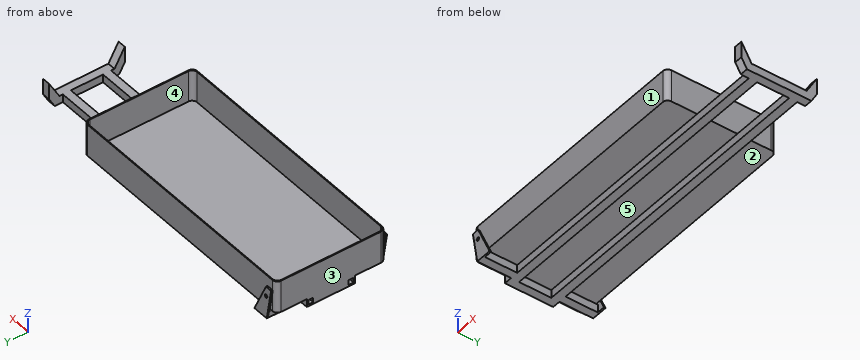
```python
from build123d import *

# Parameters (mm, degrees)
F0_W          = 990.6
F0_H          = 127
F1_DEPTH      = 431.8
F2_R          = 19.05
F4_DEPTH      = 123.825
F5_W          = 31.75
F5_H          = 31.75
F5_W_2        = 19.05
F5_H_2        = 19.05
F6_DEPTH      = 762
F6_DEPTH_BACK = 495.3
F7_W          = 31.75
F7_H          = 31.75
F7_W_2        = 19.0499997139
F7_H_2        = 19.0499997139
F8_DEPTH      = 127
F10_W         = 31.75
F10_H         = 31.75
F10_W_2       = 19.05
F10_H_2       = 19.05
F11_DEPTH     = 127
F12_W         = 31.75
F12_H         = 31.75
F12_W_2       = 19.0499814987
F12_H_2       = 19.0499814987
F13_DEPTH     = 127
F15_R         = 6.35
F16_DEPTH     = 6.35
F18_R         = 6.35
F19_DEPTH     = 6.35
F22_DEPTH     = 31.75


with BuildPart() as f1:
    # F0 (on Front) → F1 (new body)
    with BuildSketch(Plane.XZ):
        Rectangle(F0_W, F0_H)
    extrude(amount=F1_DEPTH)

    # F2
    f2_edges = [f1.edges().sort_by_distance(p)[0] for p in [
        (495.3, -431.8, 0),
        (495.3, 0, 0),
        (-495.3, -431.8, 0),
        (-495.3, 0, 0),
    ]]
    fillet(f2_edges, radius=F2_R)

    # F3 (on face) → F4 (cut)
    with BuildSketch(Plane.XY.offset(63.5)):
        with BuildLine():
            ThreePointArc((492.125, -22.225), (486.5453841816, -8.7546158184), (473.075, -3.175))
            Line((473.075, -3.175), (-473.075, -3.175))
            ThreePointArc((-473.075, -3.175), (-486.5453841816, -8.7546158184), (-492.125, -22.225))
            Line((-492.125, -22.225), (-492.125, -409.575))
            ThreePointArc((-492.125, -409.575), (-486.5453841816, -423.0453841816), (-473.075, -428.625))
            Line((-473.075, -428.625), (473.075, -428.625))
            ThreePointArc((473.075, -428.625), (486.5453841816, -423.0453841816), (492.125, -409.575))
            Line((492.125, -409.575), (492.125, -22.225))
        make_face()
    extrude(amount=-F4_DEPTH, mode=Mode.SUBTRACT)

    # F5 (on Right) → F6 (join, two sides)
    with BuildSketch(Plane.YZ) as f6_sk:
        with Locations((-295.275, -79.375)):
            Rectangle(F5_W, F5_H)
        with Locations((-295.275, -79.375)):
            Rectangle(F5_W_2, F5_H_2, mode=Mode.SUBTRACT)
        with Locations((-136.525, -79.375)):
            Rectangle(F5_W, F5_H)
        with Locations((-136.525, -79.375)):
            Rectangle(F5_W_2, F5_H_2, mode=Mode.SUBTRACT)
    extrude(amount=F6_DEPTH)
    extrude(f6_sk.sketch, amount=-F6_DEPTH_BACK)

    # F7 (on face) → F8 (join)
    with BuildSketch(Plane.XZ.offset(152.4)):
        with Locations((-479.425, -79.375)):
            Rectangle(F7_W, F7_H)
        with Locations((-479.425, -79.375)):
            Rectangle(F7_W_2, F7_H_2, mode=Mode.SUBTRACT)
    extrude(amount=F8_DEPTH)

    # F10 (on face) → F11 (join)
    with BuildSketch(Plane.XZ.offset(311.15)):
        with Locations((-447.675, -79.375)):
            Rectangle(F10_W, F10_H)
        with Locations((-447.675, -79.375)):
            Rectangle(F10_W_2, F10_H_2, mode=Mode.SUBTRACT)
    extrude(amount=F11_DEPTH)

    # F12 (on face) → F13 (join)
    with BuildSketch(Plane(origin=(0, -120.65, 0), x_dir=(-1, 0, 0), z_dir=(0, 1, 0))):
        with Locations((447.675, -79.375)):
            Rectangle(F12_W, F12_H)
        with Locations((447.675, -79.375)):
            Rectangle(F12_W_2, F12_H_2, mode=Mode.SUBTRACT)
    extrude(amount=F13_DEPTH)

    # F15 (on offset) → F16 (join)
    with BuildSketch(Plane.XZ.offset(438.15)):
        with BuildLine():
            Line((-485.2864735093, 28.0236670359), (-463.55, -95.25))
            Line((-463.55, -95.25), (-405.0337517073, -95.25))
            ThreePointArc((-405.0337517073, -95.25), (-402.3559838669, -93.7809262565), (-402.1562244835, -90.733187019))
            Line((-402.1562244835, -90.733187019), (-458.4162434399, 29.916812981))
            ThreePointArc((-458.4162434399, 29.916812981), (-459.5878444072, 31.2527678405), (-461.2937706637, 31.75))
            Line((-461.2937706637, 31.75), (-482.1597088935, 31.75))
            ThreePointArc((-482.1597088935, 31.75), (-484.5919000004, 30.6158506608), (-485.2864735093, 28.0236670359))
        make_face()
        with Locations((-459.8815916286, -6.35)):
            Circle(F15_R, mode=Mode.SUBTRACT)
    extrude(amount=F16_DEPTH)

    # F18 (on offset) → F19 (join)
    with BuildSketch(Plane(origin=(0, 6.35, 0), x_dir=(-1, 0, 0), z_dir=(0, 1, 0))):
        Polygon((400.05, -95.25), (463.55, -95.25), (485.94352655, 31.75), (459.2710725857, 31.75), align=None)
        with Locations((459.8815916286, -6.35)):
            Circle(F18_R, mode=Mode.SUBTRACT)
    extrude(amount=F19_DEPTH)

    # F21 (on offset) → F22 (join)
    with BuildSketch(Plane.YZ.offset(762)):
        Polygon((-324.5691289532, -63.5), (-364.8970452561, 6.35), (-364.8970452561, -57.15), (-342.9, -95.25), (-88.9, -95.25), (-66.9029547439, -57.15), (-66.9029547439, 6.35), (-107.2308710468, -63.5), align=None)
    extrude(amount=F22_DEPTH)


solid = f1.part
```
Could you check a few things on this model? Use its own coordinates, in mm. Face numbers are marked on the shaded views. A direction names the side the tool comes from. Coordinates: 2 decimals unless noted, no trailing zeros. Order: outer loops, then holes, each group sorted by start corner. A loop starts at its lowest first (then second) coordinate and runs counter-clockwise, first axis right, second up. Notation, with made-up numbers: M -20,66.5 L -10,66.5 A10 cw -10,70.5 Z; hole C 42,19 d11. An arc over 180 degrees is marked long. Use a Markdown table: item, result. Add a question column.
Q1. Which directions (+Z, -Z, +X, -X, +Y, -Y) give clear straight access to the entire face, cutting with the end or side of a thin tool? Please do the marked faces 4 and 5.
Q2. If I drill on L1, parallel to X at y = -84, z = -39.5 (3 decimals); L2, parallel to Y at x = 400, z = 39 (3 decimals); L3, parallel to Z at x = 46.5, y = -299 (3 decimals), over which ranges is the centre line in solid material (lowest first)?
Q3. I want a section at D-D on z = 46.5. List the corners of the cut face in (x, y) for me (3 decimals).
Q4. I want a section at B-B on y = -170.5. List the corners of the cut face in (x, z) for me (3 decimals), then the cut area to 3 significant figures.
Q5. We'd pull the mould along X, two halves only. Please class the marked faces 1, 2 and 3: pulls with the +X half, pulls with the -X half, needs draft (parallel to the pull), parting line crosses it, or undercut.
Q6. I want a section at A-A on x = 597.5. List the corners of the cut face in (y, z) for me.
Q7. I'm going to push flat-ended pins straight in: pin 1 (1 mm diameter, centred on x = 464.5, y = -230, fed in from +Z) (3 decimals); pin 2 (12 mm diameter, centred on x = -188.5, z = -19, fed in from +Y); pin 3 (9.5 mm diameter, centred on x = 387, z = -75, fed in from +Y). Where does each tip first touch, or does it pass through?
Q8. I want a section at C-C on x = 69.5. List the corners of the cut face in (y, z) for me (3 decimals).
Checked values:
| question | item | result |
|---|---|---|
| 1 | face 4 | +Z |
| 1 | face 5 | -Z |
| 2 | L1 | -495.3 to -492.125, 492.125 to 495.3, 762 to 793.75 |
| 2 | L2 | -431.8 to -428.625, -3.175 to 0 |
| 2 | L3 | -95.25 to -88.9, -69.85 to -60.325 |
| 3 | outline | M -495.3,-412.75 A19.05 ccw -476.25,-431.8 L 476.25,-431.8 A19.05 ccw 495.3,-412.75 L 495.3,-19.05 A19.05 ccw 476.25,0 L -476.25,0 A19.05 ccw -495.3,-19.05 Z; hole M -492.125,-409.575 A19.05 ccw -473.075,-428.625 L 473.075,-428.625 A19.05 ccw 492.125,-409.575 L 492.125,-22.225 A19.05 ccw 473.075,-3.175 L -473.075,-3.175 A19.05 ccw -492.125,-22.225 Z |
| 4 | outline | M -495.3,-95.25 L -463.55,-95.25 L -463.55,-63.5 L 495.3,-63.5 L 495.3,63.5 L 492.125,63.5 L 492.125,-60.325 L -492.125,-60.325 L -492.125,63.5 L -495.3,63.5 Z; M 762,-95.25 L 793.75,-95.25 L 793.75,-63.5 L 762,-63.5 Z; hole M -488.95,-88.9 L -469.9,-88.9 L -469.9,-69.85 L -488.95,-69.85 Z |
| 4 | area | 5,580 mm² |
| 5 | face 1 | needs draft |
| 5 | face 2 | undercut |
| 5 | face 3 | pulls with the -X half |
| 6 | outline | M -311.15,-95.25 L -279.4,-95.25 L -279.4,-63.5 L -311.15,-63.5 Z; M -152.4,-95.25 L -120.65,-95.25 L -120.65,-63.5 L -152.4,-63.5 Z; hole M -304.8,-88.9 L -285.75,-88.9 L -285.75,-69.85 L -304.8,-69.85 Z; hole M -146.05,-88.9 L -127,-88.9 L -127,-69.85 L -146.05,-69.85 Z |
| 7 | pin 1 | z = -60.325 |
| 7 | pin 2 | y = 0 |
| 7 | pin 3 | y = -120.65 |
| 8 | outline | M -431.8,-63.5 L -311.15,-63.5 L -311.15,-95.25 L -279.4,-95.25 L -279.4,-63.5 L -152.4,-63.5 L -152.4,-95.25 L -120.65,-95.25 L -120.65,-63.5 L 0,-63.5 L 0,63.5 L -3.175,63.5 L -3.175,-60.325 L -428.625,-60.325 L -428.625,63.5 L -431.8,63.5 Z; hole M -304.8,-88.9 L -285.75,-88.9 L -285.75,-69.85 L -304.8,-69.85 Z; hole M -146.05,-88.9 L -127,-88.9 L -127,-69.85 L -146.05,-69.85 Z |
